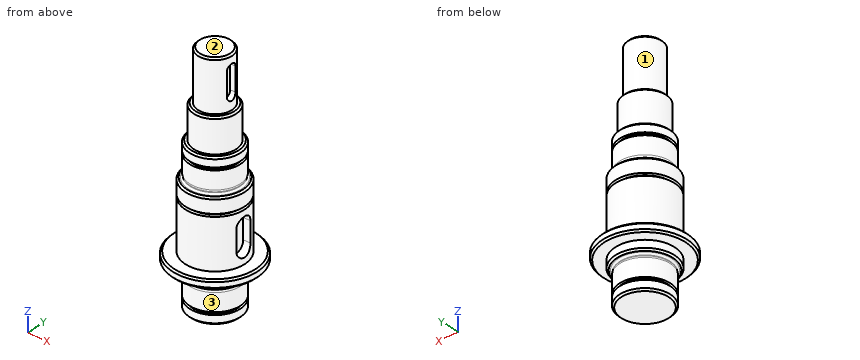
Autodesk Inventor part; units mm, degrees
ref_plane "Arbeitsebene1" through (10, 0, 0) normal (1, 0, 0) x (0, 1, 0)
ref_plane "Arbeitsebene2" through (17.5, 0, 0) normal (1, 0, 0) x (0, 1, 0)
ref_plane "XZ Plane" through (0, 0, 0) normal (0, 1, 0) x (-1, 0, 0)
sketch "Skizze1" plane through (0, 0, 0) normal (1, 0, 0) x (0, 1, 0)
  line L0 (0, 95) -> (10, 95)
  line L1 (10, 95) -> (10, 65)
  line L2 (10, 65) -> (12.5, 65)
  line L3 (12.5, 65) -> (12.5, 45)
  line L4 (12.5, 45) -> (15, 45)
  line L5 (17.5, -14.649) -> (25, -14.649)
  line L6 (25, -14.649) -> (25, -19.649)
  line L7 (25, -19.649) -> (17.5, -19.649)
  line L8 (17.5, -19.649) -> (17.5, -25)
  line L9 (15, -45) -> (0, -45)
  line L10 (0, 123) -> (0, -73)
  line L11 (-5, 0) -> (30, 0)
  line L12 (15, 45) -> (15, 39.6)
  line L13 (15, 39.6) -> (13.6, 39.6)
  line L14 (13.6, 39.6) -> (13.6, 38)
  line L15 (13.6, 38) -> (15, 38)
  line L16 (15, 38) -> (15, 27.5)
  line L17 (15, 27.5) -> (14.7, 26.3804)
  arc A0 (14.7, 26.3804) -> (14.6659, 26.1216) centre (15.6659, 26.1216) ccw
  arc A1 (14.6659, 25.8728) -> (15.7, 25) centre (15.6579, 25.9991) ccw
  line L18 (14.6659, 25.8728) -> (14.6659, 26.1216)
  line L19 (17.5, 25) -> (15.7, 25)
  line L20 (15, -45) -> (15, -39.6)
  line L21 (15, -39.6) -> (13.6, -39.6)
  line L22 (13.6, -39.6) -> (13.6, -38)
  line L23 (13.6, -38) -> (15, -38)
  line L24 (15, -38) -> (15, -27.5)
  line L25 (15, -27.5) -> (14.7341, -26.5076)
  line L26 (17.5, -25) -> (16, -25)
  line L27 (16, -25) -> (15.7, -25)
  arc A2 (15.7, -25) -> (14.7, -26) centre (15.7, -26) ccw
  arc A3 (14.7, -26.2487) -> (14.7341, -26.5076) centre (15.7, -26.2487) ccw
  line L28 (14.7, -26.2487) -> (14.7, -26)
  line L29 (17.5, 25) -> (17.5, 16.249)
  line L30 (17.5, 16.249) -> (15.5, 16.249)
  line L31 (15.5, 16.249) -> (15.5, 14.649)
  line L32 (15.5, 14.649) -> (17.5, 14.649)
  line L33 (17.5, 14.649) -> (17.5, -14.649)
  point P0 (0, 0)
  point P1 (14.6579, 24.9991)
  point P2 (14.7, -26.3804)
  point P3 (14.7, -25)
  dimension "d0" = 20
  dimension "d3" = 25
  dimension "d5" = 50
  dimension "d6" = 20
  dimension "d7" = 30
  dimension "d10" = 5
  dimension "d11" = 50
  dimension "d13" = 2.5
  dimension "d17" = 1
  dimension "d18" = 1
  dimension "d20" = 30
  dimension "d21" = 20
  dimension "d22" = 0.3
  dimension "d23" = 15
  dimension "d25" = 1.6
  dimension "d26" = 1.4
  dimension "d28" = 2.5
  dimension "d31" = 1
  dimension "d32" = 15
  dimension "d33" = 0.3
  dimension "d34" = 1
  dimension "d35" = 1.4
  dimension "d36" = 1.6
  dimension "d37" = 13
  dimension "d38" = 20
  dimension "d39" = 1.6
  dimension "d40" = 2
  dimension "d83" = 14.649
  dimension "d84" = 29.298
  dimension "d85" = 13
  dimension "d86" = 35
revolve "Umdrehung1" add sketch "Skizze1" angle 360 about axis through (0, 0, 0) along (0, 0, -1)
chamfer "Fase1" distance 1 angle 45 1 edges at (0, -10, 95) measured on face at (2.9244, -0.4018, 95)
chamfer "Fase2" distance 1 angle 45 1 edges at (0, -12.5, 65) measured on face at (-1.7949, 11.4487, 65)
chamfer "Fase3" distance 1 angle 45 1 edges at (0, -15, 45) measured on face at (-1.1966, 14.0214, 45)
chamfer "Fase4" distance 1 angle 45 1 edges at (0, -17.5, 25) measured on face at (-1.396, 16.7305, 25)
chamfer "Fase5" distance 1 angle 45 1 edges at (0, -25, -14.649) measured on face at (-1.9943, 22.2578, -14.649)
chamfer "Fase6" distance 1 angle 45 1 edges at (0, -25, -19.649) measured on face at (-3.3903, 22.0883, -19.649)
chamfer "Fase7" distance 1 angle 45 1 edges at (0, -17.5, -25) measured on face at (-1.396, 16.8305, -25)
chamfer "Fase8" distance 1 angle 45 1 edges at (0, -15, -45) measured on face at (2.9183, -2.695, -45)
ref_plane "Arbeitsebene1" through (10, 0, 0) normal (1, 0, 0) x (0, 1, 0)
sketch "Skizze2" plane through (10, 0, 0) normal (1, 0, 0) x (0, 1, 0)
  line L0 (0, 87) -> (0, 73) construction
  line L1 (-3, 87) -> (-3, 73)
  line L2 (3, 73) -> (3, 87)
  arc A0 (3, 87) -> (-3, 87) centre (0, 87) ccw
  arc A1 (-3, 73) -> (3, 73) centre (0, 73) ccw
  line L3 (-9, 95) -> (9, 95)
  point P0 (0, 0)
  point P1 (0, 80)
  dimension "d68" = 20
  dimension "d69" = 15
  dimension "d70" = 6
extrude "Extrusion1" cut sketch "Skizze2" against normal blind 3.55
ref_plane "Arbeitsebene2" through (17.5, 0, 0) normal (1, 0, 0) x (0, 1, 0)
sketch "Skizze3" plane through (17.5, 0, 0) normal (1, 0, 0) x (0, 1, 0)
  line L0 (0, 6) -> (0, -6) construction
  line L1 (-5, 6) -> (-5, -6)
  line L2 (5, -6) -> (5, 6)
  arc A0 (5, 6) -> (-5, 6) centre (0, 6) ccw
  arc A1 (-5, -6) -> (5, -6) centre (0, -6) ccw
  line L3 (-7, 0) -> (7, 0)
  point P0 (0, 0)
  point P1 (0, 0)
  dimension "d74" = 22
  dimension "d75" = 10
extrude "Extrusion2" cut sketch "Skizze3" against normal blind 5 and the other way blind 1.45
equation "\"dd0\" = 6"
equation "\"dd1\" = 4"
properties part number "AbtriebswelleZahnrad 2" material "Stahl, Legierung"
Input: part model. Units: mm. Frame: model coordinates. Face numbers are marked on the shaded views. A direction names the side the tool comes from. Coordinates: 2 decimals unless noted, no trailing zeros. Loops run counter-clockwise (first coordinate to the right, second up) from the corner with the lowest first, then second, coordinate; pieces in that order, holes last. Notation, with made-up numbers: (21, -31) - (79, -31) arc R27 ccw to (79, 5) - close; hole circle Ø7 at (-13, 65.5). An arc over 180 degrees is marked (long way). Answer in a Markdown table with one row per item. Add a question column.
Item 1: Contact query for flat-ended pins moving along their axis: P1, Ø1.5, axis at x = -15, z = 14, coming from the +Y side; P2, Ø12, axis at x = 18.5, y = 11.5, coming from the -Z side; P3, Ø2, axis at x = 14.5, z = 1, coming from the -Y side. Output: stop coordinate, or through.
Item 2: Section query B-B on z = 19.5. Return the cut outline in (x, y), then the cut area to 3 significant figures.
Item 3: Line query: line 1 along Z through (x, y) = (12, -11); line 2 along Z through (x, y) = (3.5, 19.5); line 3 along Z through (x, y) = (-6, 13). Output: solid intervals per line, ascending. Write a range as [from, to].
Item 4: Access query for the marked faces 1, 2 and 3. Directions: +Z, -Z, +X, -X, +Y, -Y. A direction counts if a zero-diameter tool reaches every point of the face in a straight line with its end or side. Return the directions, or none.
Item 5: Section query A-A on z = 82. Return the cut outline in (x, y).
Item 6: Section query C-C on z = -2. Return the cut outline in (x, y), then the cut area to 3 significant figures.
Recorded:
| question | item | result |
|---|---|---|
| 1 | P1 | y = 10.16 |
| 1 | P2 | z = -25 |
| 1 | P3 | y = -11.14 |
| 2 | outline | circle Ø35 at (0, 0) |
| 2 | area | 962 mm^2 |
| 3 | line 1 | [-25, 14.65], [16.25, 25] |
| 3 | line 2 | [-19.65, -14.65] |
| 3 | line 3 | [-44.68, -39.6], [-38, 38], [39.6, 44.68] |
| 4 | face 1 | +Z |
| 4 | face 2 | +Z, +X, -X, +Y, -Y |
| 4 | face 3 | -Z |
| 5 | outline | (6.45, -3) - (6.45, 3) - (9.54, 3) arc R10 ccw (long way) to (9.54, -3) - close |
| 6 | outline | (12.5, -5) - (12.5, 5) - (16.77, 5) arc R17.5 ccw (long way) to (16.77, -5) - close |
| 6 | area | 915 mm^2 |
